Could you check a few things on this model? Use its own coordinates, in mm. A direction names the side the tool comes from. Coordinates: 2 decimals unless noted, no trailing zeros. Write each loop counter-clockwise with the first axis right and the second up, starting at its lowest first coordinate (ties: lowest second). Pieces come first, ordered by that corner, then holes.
Item 1: Which directions (+Z, -Z, +X, -X, +Y, -Y) give clear straight access to the entire face, cutting with the end or side of a thin tool? Please do faces 1 (the cylindrical face through (69.199, 17.235, 3.007)), 2 (the flat face through (2, 19, 78)), 3 (the flat face through (2.5, 20, 70)), 4 (the flat face through (3.5, 19, 75)).
Item 2: Thinking about a two-plate mould opening in Z: for faces 5 (the flat face through (73, 18, 2.5)), 6 (the flat face through (45, 13, 48)), 7 (the cylindrical face through (2, 19, 73)), which applies, +Z half, -Z half, draft (parallel to the pull), parting line (faces both ways), or undercut?
Item 3: I want a section at C-C on x = 38. Please give me the cut outline in (y, z).
Item 4: I want a section at D-D on z = 15. Please give me the cut outline in (x, y), then the cut area to 3 significant figures.
Item 5: For P1, Ø1.5, axis at y = 21, z = 11.5, coming from the -X side; P2, Ø3, axis at x = 70.5, y = 20.5, coming from the +Z side; P3, Ø6, axis at y = 18, z = 71, coming from the +X side; P4, Ø2.5, axis at x = 71.5, y = 19, coming from the -Z side, each with a flat end and sliding along its axis, tell me the tip position at first contact or that it passes through.
Item 6: If I drill on probe 1 along Y at (x, z) = (2.05, 71.5); probe 2 along X at (y, z) = (23.5, 75.5); probe 3 along Y at (x, z) = (71, 2), over which ranges is the centre line in solid material (lowest first)?
Item 7: I want a section at B-B on z = 71.5. Please give me the cut outline in (x, y), then the cut area to 3 significant figures.
Item 8: I want a section at A-A on x = 71.5. Please give me the cut outline in (y, z), then the cut area to 3 significant figures.
from build123d import *

# Parameters (mm, degrees)
SKETCH1_R                   = 68
SKETCH1_R_2                 = 65
BOSS_EXTRUDE1_DEPTH         = 25
BOSS_EXTRUDE2_START         = -0.090133
SKETCH2_W                   = 7
SKETCH2_H                   = 50
BOSS_EXTRUDE2_DEPTH         = 10.090133
SKETCH3_W                   = 2
SKETCH3_H                   = 50
CUT_EXTRUDE1_DEPTH          = 10
CIRPATTERN2_COUNT           = 4
SKETCH7_R                   = 2.9
CUT_EXTRUDE4_DEPTH          = 1
CUT_EXTRUDE5_DEPTH          = 1
SKETCH9_R                   = 1.5
CUT_EXTRUDE6_DEPTH          = 115.844460032
CIRPATTERN3_COUNT           = 4
CIRPATTERN3_COPY_1_SKETCH_R = 2.9
CIRPATTERN3_COPY_1_DEPTH    = 1
CIRPATTERN3_COPY_2_SKETCH_R = 2.9
CIRPATTERN3_COPY_2_DEPTH    = 1
CIRPATTERN3_COPY_3_SKETCH_R = 2.9
CIRPATTERN3_COPY_3_DEPTH    = 1
CIRPATTERN3_COPY_4_DEPTH    = 1
CIRPATTERN3_COPY_5_DEPTH    = 1
CIRPATTERN3_COPY_6_DEPTH    = 1
CIRPATTERN3_COPY_7_SKETCH_R = 1.5
CIRPATTERN3_COPY_7_DEPTH    = 115.844460032
CIRPATTERN3_COPY_8_SKETCH_R = 1.5
CIRPATTERN3_COPY_8_DEPTH    = 115.844460032
CIRPATTERN3_COPY_9_SKETCH_R = 1.5
CIRPATTERN3_COPY_9_DEPTH    = 115.844460032
SKETCH10_W                  = 172.322225858
SKETCH10_H                  = 181.395343574
CUT_EXTRUDE7_DEPTH          = 13
CUT_EXTRUDE7_DEPTH_BACK     = 114.106144837
SKETCH4_W                   = 204.796424039
SKETCH4_H                   = 80.613482063
CUT_EXTRUDE2_DEPTH          = 114.106144837
SKETCH5_W                   = 133.005640426
SKETCH5_H                   = 101.362408315
CUT_EXTRUDE3_DEPTH          = 114.106144837
SKETCH11_W                  = 1
SKETCH11_H                  = 12
CUT_EXTRUDE8_DEPTH          = 107.456563912
CUT_EXTRUDE8_DEPTH_BACK     = 107.456563912
SKETCH12_W                  = 1
SKETCH12_H                  = 12
CUT_EXTRUDE9_DEPTH          = 10


with BuildPart() as part:
    # Sketch1 → Boss-Extrude1 (new, symmetric)
    with BuildSketch(Plane(origin=(0, 0, 0), x_dir=(1, 0, 0), z_dir=(0, 1, 0))):
        with Locations(Location((0, 0, 0), (0, 0, 270))):
            Circle(SKETCH1_R)
        with Locations(Location((0, 0, 0), (0, 0, 270))):
            Circle(SKETCH1_R_2, mode=Mode.SUBTRACT)
    extrude(amount=BOSS_EXTRUDE1_DEPTH, both=True)

    # Sketch2 → Boss-Extrude2 (add)
    with BuildSketch(Plane(origin=(68, 0, 0), x_dir=(0, 0, -1), z_dir=(1, 0, 0)).offset(BOSS_EXTRUDE2_START)):
        Rectangle(SKETCH2_W, SKETCH2_H)
    boss_extrude2 = extrude(amount=BOSS_EXTRUDE2_DEPTH)

    # Sketch3 → Cut-Extrude1 (cut)
    with BuildSketch(Plane(origin=(78, 0, 0), x_dir=(0, 0, -1), z_dir=(1, 0, 0))):
        Rectangle(SKETCH3_W, SKETCH3_H)
    cut_extrude1 = extrude(amount=-CUT_EXTRUDE1_DEPTH, mode=Mode.SUBTRACT)

    # CirPattern2: Boss-Extrude2, Cut-Extrude1 ×4 about axis
    cirpattern2_axis = Axis((0, 0, 0), (0, 1, 0))
    add([boss_extrude2.rotate(cirpattern2_axis, i * 360 / CIRPATTERN2_COUNT) for i in range(1, CIRPATTERN2_COUNT)])
    add([cut_extrude1.rotate(cirpattern2_axis, i * 360 / CIRPATTERN2_COUNT) for i in range(1, CIRPATTERN2_COUNT)], mode=Mode.SUBTRACT)

    # Sketch7 → Cut-Extrude4 (cut)
    with BuildSketch(Plane.XY.offset(3.5)):
        with Locations((71.5, 19)):
            Circle(SKETCH7_R)
    cut_extrude4 = extrude(amount=-CUT_EXTRUDE4_DEPTH, mode=Mode.SUBTRACT)

    # Sketch8 → Cut-Extrude5 (cut)
    with BuildSketch(Plane(origin=(0, 0, -3.5), x_dir=(-1, 0, 0), z_dir=(0, 0, -1))):
        Polygon((-69.91228676, 16.25), (-68.324573519, 19), (-69.91228676, 21.75), (-73.08771324, 21.75), (-74.675426481, 19), (-73.08771324, 16.25), align=None)
    cut_extrude5 = extrude(amount=-CUT_EXTRUDE5_DEPTH, mode=Mode.SUBTRACT)

    # Sketch9 → Cut-Extrude6 (cut, through all)
    with BuildSketch(Plane.XY.offset(2.5)):
        with Locations((71.5, 19)):
            Circle(SKETCH9_R)
    cut_extrude6 = extrude(amount=-CUT_EXTRUDE6_DEPTH, mode=Mode.SUBTRACT)

    # Mirror1: Cut-Extrude4, Cut-Extrude5, Cut-Extrude6 across plane
    add(cut_extrude4.mirror(Plane.ZX), mode=Mode.SUBTRACT)
    add(cut_extrude5.mirror(Plane.ZX), mode=Mode.SUBTRACT)
    add(cut_extrude6.mirror(Plane.ZX), mode=Mode.SUBTRACT)

    # CirPattern3: Cut-Extrude4, Cut-Extrude5, Cut-Extrude6 ×4 about axis
    cirpattern3_axis = Axis((0, 0, 0), (0, 1, 0))
    add([cut_extrude4.rotate(cirpattern3_axis, i * 360 / CIRPATTERN3_COUNT) for i in range(1, CIRPATTERN3_COUNT)], mode=Mode.SUBTRACT)
    add([cut_extrude5.rotate(cirpattern3_axis, i * 360 / CIRPATTERN3_COUNT) for i in range(1, CIRPATTERN3_COUNT)], mode=Mode.SUBTRACT)
    add([cut_extrude6.rotate(cirpattern3_axis, i * 360 / CIRPATTERN3_COUNT) for i in range(1, CIRPATTERN3_COUNT)], mode=Mode.SUBTRACT)

    # CirPattern3 copy 1 sketch → CirPattern3 copy 1 (cut)
    with BuildSketch(Plane(origin=(3.5, 0, 0), x_dir=(0, 0, -1), z_dir=(1, 0, 0))):
        with Locations((71.5, -19)):
            Circle(CIRPATTERN3_COPY_1_SKETCH_R)
    extrude(amount=-CIRPATTERN3_COPY_1_DEPTH, mode=Mode.SUBTRACT)

    # CirPattern3 copy 2 sketch → CirPattern3 copy 2 (cut)
    with BuildSketch(Plane(origin=(0, 0, -3.5), x_dir=(-1, 0, 0), z_dir=(0, 0, -1))):
        with Locations((71.5, -19)):
            Circle(CIRPATTERN3_COPY_2_SKETCH_R)
    extrude(amount=-CIRPATTERN3_COPY_2_DEPTH, mode=Mode.SUBTRACT)

    # CirPattern3 copy 3 sketch → CirPattern3 copy 3 (cut)
    with BuildSketch(Plane.ZY.offset(3.5)):
        with Locations((71.5, -19)):
            Circle(CIRPATTERN3_COPY_3_SKETCH_R)
    extrude(amount=-CIRPATTERN3_COPY_3_DEPTH, mode=Mode.SUBTRACT)

    # CirPattern3 copy 4 sketch → CirPattern3 copy 4 (cut)
    with BuildSketch(Plane.ZY.offset(3.5)):
        Polygon((-69.91228676, -16.25), (-68.324573519, -19), (-69.91228676, -21.75), (-73.08771324, -21.75), (-74.675426481, -19), (-73.08771324, -16.25), align=None)
    extrude(amount=-CIRPATTERN3_COPY_4_DEPTH, mode=Mode.SUBTRACT)

    # CirPattern3 copy 5 sketch → CirPattern3 copy 5 (cut)
    with BuildSketch(Plane.XY.offset(3.5)):
        Polygon((-69.91228676, -16.25), (-68.324573519, -19), (-69.91228676, -21.75), (-73.08771324, -21.75), (-74.675426481, -19), (-73.08771324, -16.25), align=None)
    extrude(amount=-CIRPATTERN3_COPY_5_DEPTH, mode=Mode.SUBTRACT)

    # CirPattern3 copy 6 sketch → CirPattern3 copy 6 (cut)
    with BuildSketch(Plane(origin=(3.5, 0, 0), x_dir=(0, 0, -1), z_dir=(1, 0, 0))):
        Polygon((-69.91228676, -16.25), (-68.324573519, -19), (-69.91228676, -21.75), (-73.08771324, -21.75), (-74.675426481, -19), (-73.08771324, -16.25), align=None)
    extrude(amount=-CIRPATTERN3_COPY_6_DEPTH, mode=Mode.SUBTRACT)

    # CirPattern3 copy 7 sketch → CirPattern3 copy 7 (cut, through all)
    with BuildSketch(Plane(origin=(2.5, 0, 0), x_dir=(0, 0, -1), z_dir=(1, 0, 0))):
        with Locations((71.5, -19)):
            Circle(CIRPATTERN3_COPY_7_SKETCH_R)
    extrude(amount=-CIRPATTERN3_COPY_7_DEPTH, mode=Mode.SUBTRACT)

    # CirPattern3 copy 8 sketch → CirPattern3 copy 8 (cut, through all)
    with BuildSketch(Plane(origin=(0, 0, -2.5), x_dir=(-1, 0, 0), z_dir=(0, 0, -1))):
        with Locations((71.5, -19)):
            Circle(CIRPATTERN3_COPY_8_SKETCH_R)
    extrude(amount=-CIRPATTERN3_COPY_8_DEPTH, mode=Mode.SUBTRACT)

    # CirPattern3 copy 9 sketch → CirPattern3 copy 9 (cut, through all)
    with BuildSketch(Plane.ZY.offset(2.5)):
        with Locations((71.5, -19)):
            Circle(CIRPATTERN3_COPY_9_SKETCH_R)
    extrude(amount=-CIRPATTERN3_COPY_9_DEPTH, mode=Mode.SUBTRACT)

    # Sketch10 → Cut-Extrude7 (cut, two sides)
    with BuildSketch(Plane(origin=(0, 0, 0), x_dir=(1, 0, 0), z_dir=(0, 1, 0))) as cut_extrude7_sk:
        with Locations((0.161152427, 1.352018999)):
            Rectangle(SKETCH10_W, SKETCH10_H)
    extrude(amount=CUT_EXTRUDE7_DEPTH, mode=Mode.SUBTRACT)
    extrude(cut_extrude7_sk.sketch, amount=-CUT_EXTRUDE7_DEPTH_BACK, mode=Mode.SUBTRACT)

    # Sketch4 → Cut-Extrude2 (cut, through all)
    with BuildSketch(Plane.XY):
        with Locations((-0.265516435, -0.614198292)):
            Rectangle(SKETCH4_W, SKETCH4_H)
    extrude(amount=-CUT_EXTRUDE2_DEPTH, mode=Mode.SUBTRACT)

    # Sketch5 → Cut-Extrude3 (cut, through all)
    with BuildSketch(Plane(origin=(0, 0, 0), x_dir=(0, 0, -1), z_dir=(1, 0, 0))):
        with Locations((-14.085466414, 0.839605882)):
            Rectangle(SKETCH5_W, SKETCH5_H)
    extrude(amount=-CUT_EXTRUDE3_DEPTH, mode=Mode.SUBTRACT)

    # Sketch11 → Cut-Extrude8 (cut, two sides)
    with BuildSketch(Plane(origin=(68, 0, 0), x_dir=(0, 0, -1), z_dir=(1, 0, 0))) as cut_extrude8_sk:
        with Locations((-0.5, 19)):
            Rectangle(SKETCH11_W, SKETCH11_H)
    extrude(amount=CUT_EXTRUDE8_DEPTH, mode=Mode.SUBTRACT)
    extrude(cut_extrude8_sk.sketch, amount=-CUT_EXTRUDE8_DEPTH_BACK, mode=Mode.SUBTRACT)

    # Sketch12 → Cut-Extrude9 (cut)
    with BuildSketch(Plane.XY.offset(68)):
        with Locations((0.5, 19)):
            Rectangle(SKETCH12_W, SKETCH12_H)
    extrude(amount=-CUT_EXTRUDE9_DEPTH, mode=Mode.SUBTRACT)


solid = part.part
Response values:
1. face 1: +Z
1. face 2: +Z, +X, -X, +Y, -Y
1. face 3: +X
1. face 4: +Z, +X, +Y, -Y
2. face 5: +Z half
2. face 6: draft
2. face 7: undercut
3. outline: (13, 52.74) - (25, 52.74) - (25, 56.39) - (13, 56.39) - close
4. outline: (63.25, 13) - (66.32, 13) - (66.32, 25) - (63.25, 25) - close
4. area: 37.0 mm2
5. P1: stops at x = 63.84
5. P2: stops at z = 3.5
5. P3: stops at x = 3.5
5. P4: passes through
6. probe 1: y = 13 to 17.5, 20.5 to 25
6. probe 2: x = 1 to 3.5
6. probe 3: y = 13 to 17.59, 20.41 to 25
7. outline: (1, 13) - (3.5, 13) - (3.5, 16.25) - (2.5, 16.25) - (2.5, 17.5) - (1, 17.5) - close; (1, 20.5) - (2.5, 20.5) - (2.5, 21.75) - (3.5, 21.75) - (3.5, 25) - (1, 25) - close
7. area: 20.0 mm2
8. outline: (13, 1) - (17.5, 1) - (17.5, 2.5) - (16.1, 2.5) - (16.1, 3.5) - (13, 3.5) - close; (20.5, 1) - (25, 1) - (25, 3.5) - (21.9, 3.5) - (21.9, 2.5) - (20.5, 2.5) - close
8. area: 19.7 mm2
